from build123d import *

# Parameters (mm, degrees)
SCHIZZO2_R                   = 2.54
SCHIZZO2_W                   = 11.43
SCHIZZO2_H                   = 29.21
ESTRUSIONE_ESTRUSIONE1_DEPTH = 1.25


with BuildPart() as part:
    # Schizzo2 → Estrusione-Estrusione1 (new, symmetric)
    with BuildSketch(Plane(origin=(0, 0, 0), x_dir=(1, 0, 0), z_dir=(0, 1, 0))):
        Polygon((-18, 15), (-16, 15), (-16, -15), (-18, -15), (-18, -25), (20, -25), (20, -15), (18, -15), (18, 15), (20, 15), (20, 25), (-18, 25), align=None)
        with Locations(Location((1, 18.985370086, 0), (0, 0, 270))):
            Circle(SCHIZZO2_R, mode=Mode.SUBTRACT)
        with Locations(Location((1, -18.985370086, 0), (0, 0, 270))):
            Circle(SCHIZZO2_R, mode=Mode.SUBTRACT)
        Rectangle(SCHIZZO2_W, SCHIZZO2_H, mode=Mode.SUBTRACT)
    extrude(amount=ESTRUSIONE_ESTRUSIONE1_DEPTH, both=True)


solid = part.part
Input: part model. Units: mm. Frame: model coordinates. A direction names the side the tool comes from. Coordinates: 2 decimals unless noted, no trailing zeros. Write each loop counter-clockwise with the first axis right and the second up, starting at its lowest first coordinate (ties: lowest second). Pieces come first, ordered by that corner, then holes. Notation, with made-up numbers: M 68.5,-0.75 L 101.5,-0.75 A24 ccw 101.5,15.25 Z; hole C 60,57 d2. An arc over 180 degrees is marked long. Answer as a JSON object with one key per item and string values. Group by question number.
(1) Section B-B on y = -0.05. Output: boundary loops of the cut face in (x, z) (3 decimals).
(2) Set-up query: faces 4 (the face through (9, 1.25, 0)), 5 (the face through (-17, 0, 15)), 6 (the face through (19, 0, 15)), 7 (the face through (1, 0, 25)), 8 (the face through (0, 0, 14.605)). Return all of +Z, -Z, +X, -X, +Y, -Y with unobstructed straight access to the full face (end or side cutting, diameter ignored); none if empty.
(3) Ray query, line 1 along X through (y, z) = (-0.1, -13) (3 decimals); line 2 along Z through (x, y) = (-4.5, 1.1) (3 decimals); line 3 along X through (y, z) = (-0.3, -18.5). Return the intervals inside material, ascending. Write a range as [from, to].
(4) Section D-D on z = -19. Output: boundary loops of the cut face in (x, y).
(5) Mould query, pull axis X, two halves, no side actions, for faces 1 (the face through (-16, 0, 0)), 2 (the face through (20, 0, -20)), 3 (the face through (5.715, 0, 0)). Classes: pulls with the +X half, pulls with the -X half, needs draft (parallel to the pull), parting line crosses it, or undercut.
(6) Section A-A on x = 1. Output: boundary loops of the cut face in (y, z) (3 decimals), plus the area to 3 significant figures.
(7) Contact query for flat-ended pins moving along their axis: P1, Ø0.8, axis at y = -0.5, z = 5, coming from the +X side; P2, Ø1.2, axis at y = 0, z = -6, coming from the -X side. Output: stop coordinate, or through.
(8) Section C-C on z = -9. Output: boundary loops of the cut face in (x, y) (3 decimals), plus the area to 3 significant figures.
Result set:
{
 "1": {"outline": "M -18,-25 L 20,-25 L 20,-15 L 18,-15 L 18,15 L 20,15 L 20,25 L -18,25 L -18,15 L -16,15 L -16,-15 L -18,-15 Z; hole M -5.715,-14.605 L 5.715,-14.605 L 5.715,14.605 L -5.715,14.605 Z; hole C 1,-18.985 d5.08; hole C 1,18.985 d5.08"},
 "2": {"face 4": "+Z, -Z, +X, -X, +Y", "face 5": "-X, +Y, -Y", "face 6": "+X, +Y, -Y", "face 7": "+Z, +X, -X, +Y, -Y", "face 8": "+Y, -Y"},
 "3": {"line 1": "x = [-16, -5.715], [5.715, 18]", "line 2": "z = [-25, -14.605], [14.605, 25]", "line 3": "x = [-18, -1.49], [3.49, 20]"},
 "4": {"outline": "M -18,-1.25 L -1.54,-1.25 L -1.54,1.25 L -18,1.25 Z; M 3.54,-1.25 L 20,-1.25 L 20,1.25 L 3.54,1.25 Z"},
 "5": {"face 1": "pulls with the -X half", "face 2": "pulls with the +X half", "face 3": "undercut"},
 "6": {"outline": "M -1.25,-25 L 1.25,-25 L 1.25,-21.525 L -1.25,-21.525 Z; M -1.25,-16.445 L 1.25,-16.445 L 1.25,-14.605 L -1.25,-14.605 Z; M -1.25,14.605 L 1.25,14.605 L 1.25,16.445 L -1.25,16.445 Z; M -1.25,21.525 L 1.25,21.525 L 1.25,25 L -1.25,25 Z", "area": "26.6 mm2"},
 "7": {"P1": "stops at x = 18", "P2": "stops at x = -16"},
 "8": {"outline": "M -16,-1.25 L -5.715,-1.25 L -5.715,1.25 L -16,1.25 Z; M 5.715,-1.25 L 18,-1.25 L 18,1.25 L 5.715,1.25 Z", "area": "56.4 mm2"}
}
